Part model, mm, in its own coordinate system. A direction names the side the tool comes from. Coordinates: 2 decimals unless noted, no trailing zeros. Order: outer loops, then holes, each group sorted by start corner. A loop starts at its lowest first (then second) coordinate and runs counter-clockwise, first axis right, second up.
from build123d import *

# Parameters (mm, degrees)
BOSS_EXTRU_1_DEPTH      = 12
ESQUISSE2_R             = 2.5
ENL_V_MAT_EXTRU_1_DEPTH = 84.578466126
ENL_V_MAT_EXTRU_2_DEPTH = 88.774483764
CONG_1_R                = 6


with BuildPart() as part:
    # Esquisse1 → Boss.-Extru.1 (new body)
    with BuildSketch(Plane(origin=(0, 0, 0), x_dir=(1, 0, 0), z_dir=(0, 1, 0))):
        Polygon((-32.2, 27.00676783), (-32.2, 18.895405671), (-37.2, 27.00676783), (-37.2, 45), (37.2, 45), (37.2, 27.00676783), (32.2, 18.895405671), (32.2, 0), (27.2, 0), (27.2, 18.895405671), (32.2, 27.00676783), (32.2, 40), (-32.2, 40), align=None)
        Polygon((-32.2, 27.00676783), (-27.2, 18.895405671), (-27.2, 0), (-32.2, 0), (-32.2, 18.895405671), align=None)
    extrude(amount=BOSS_EXTRU_1_DEPTH)

    # Esquisse2 → Enlèv. mat.-Extru.1 (cut, through all)
    with BuildSketch(Plane.ZY.offset(32.2)):
        with Locations((-6, 6)):
            Circle(ESQUISSE2_R)
    extrude(amount=-ENL_V_MAT_EXTRU_1_DEPTH, mode=Mode.SUBTRACT)

    # Esquisse5 → Enlèv. mat.-Extru.2 (cut, through all)
    with BuildSketch(Plane.ZY.offset(37.2)):
        with BuildLine():
            Line((-37.247636958, 7.6), (-29.765898702, 7.6))
            ThreePointArc((-29.765898702, 7.6), (-28.165898702, 6), (-29.765898702, 4.4))
            Line((-29.765898702, 4.4), (-37.247636958, 4.4))
            ThreePointArc((-37.247636958, 4.4), (-38.847636958, 6), (-37.247636958, 7.6))
        make_face()
    extrude(amount=-ENL_V_MAT_EXTRU_2_DEPTH, mode=Mode.SUBTRACT)

    # Congé1
    cong_1_edges = [part.edges().sort_by_distance(p)[0] for p in [
        (-29.7, 0, 0),
        (-29.7, 12, 0),
        (29.7, 0, 0),
        (29.7, 12, 0),
    ]]
    fillet(cong_1_edges, radius=CONG_1_R - 0.0001)  # a hair under: the kernel refuses the full size


solid = part.part
Q1. Wall check: line 1 along Y through (x, z) = (28.75, -6); line 2 along X through (y, z) = (9.5, -35); line 3 along X through (y, z) = (11.25, -6.5). Give the ranges that are in metal, low to high.
Results list:
line 1: y = 0 to 3.5, 8.5 to 12
line 2: x = -37.2 to -32.2, 32.2 to 37.2
line 3: x = -32.2 to -27.2, 27.2 to 32.2
Q2. Cut at A-A on x = -28.5. Count the separate pieces of the cut face and the enclosed holes in it, and give its area (3 significant figures).
Results list:
separate pieces: 2
enclosed holes: 1
area: 277 mm2
Q3. Mould opens along Y. For faces 1 (the face through (29.665, 10.289, -1.804)), 2 (the face through (34.665, 6.035, -28.166)), 3 (the face through (-32.2, 6, -9)), 4 (the face through (-34.735, 6.035, -28.166)) say: pulls with the +Y half, pulls with the -Y half, needs draft (parallel to the pull), parting line crosses it, or undercut.
Results list:
face 1: pulls with the +Y half
face 2: undercut
face 3: needs draft
face 4: undercut
Q4. Cut at C-C on z = -20.5. Write the cut outline in (x, y).
Results list:
outline: (-33.19, 0) - (-28.19, 0) - (-28.19, 12) - (-33.19, 12) - close; (28.19, 0) - (33.19, 0) - (33.19, 12) - (28.19, 12) - close
Q5. Cut at D-D on x = 24. Write the cut outline in (y, z).
Results list:
outline: (0, -45) - (12, -45) - (12, -40) - (0, -40) - close
Q6. Which spindle directions (+Z, -Z, +X, -X, +Y, -Y) get a long thin tool onto all of the face, cutting with end or side? Do faces 5 (the face through (32.2, 3, -33)), 6 (the face through (35, 7.6, -34)), 7 (the face through (32.2, 6, -10)). Say none if no direction does.
Results list:
face 5: +Y, -Y
face 6: +X, -X
face 7: +Z, +X, +Y, -Y
Q7. Cut at B-B on z = -34. Write the cut outline in (x, y), and give its area (3 significant figures).
Results list:
outline: (-37.2, 0) - (-32.2, 0) - (-32.2, 4.4) - (-37.2, 4.4) - close; (-37.2, 7.6) - (-32.2, 7.6) - (-32.2, 12) - (-37.2, 12) - close; (32.2, 0) - (37.2, 0) - (37.2, 4.4) - (32.2, 4.4) - close; (32.2, 7.6) - (37.2, 7.6) - (37.2, 12) - (32.2, 12) - close
area: 88.0 mm2
Q8. Pin check, flat tips, straight feed: pin 1 Ø6 at (y, z) = (6, -6) entering from +X; pin 2 Ø4 at (x, y) = (20.5, 8.5) entering from +Z. Stop position of each tip, or through.
Results list:
pin 1: stops at x = 32.2
pin 2: stops at z = -40
